from build123d import *

# Parameters (mm, degrees)
F1_DEPTH = 5
F3_D     = 6.6


with BuildPart() as f1:
    # F0 (on Front) → F1 (new body)
    with BuildSketch(Plane.XZ):
        Polygon((-250, 300), (-310, 300), (-310, -300), (310, -300), (310, -100), align=None)
    extrude(amount=F1_DEPTH)

    # F3 (through all)
    with Locations(Plane.XZ.offset(5)):
        with Locations((-125, -285), (0, -285), (125, -285)):
            Hole(F3_D / 2)


solid = f1.part
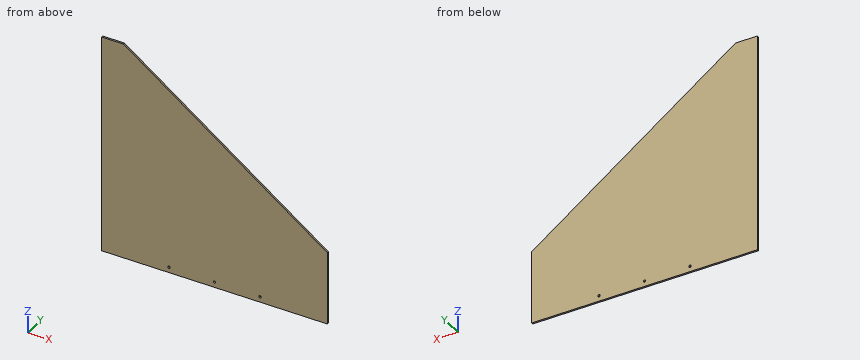
CAD build for the part. Positions are in the model's coordinates, mm. Round coordinates to 2 decimals unless told otherwise and drop trailing zeros. Loops run counter-clockwise (first coordinate to the right, second up) from the corner with the lowest first, then second, coordinate; pieces in that order, holes last.
(1) Wall check: line 1 along X through (y, z) = (-3.05, -285); line 2 along Z through (x, y) = (0, -2.7); line 3 along Z through (x, y) = (125, -2.2). Give the ranges that are in metal, low to high.
(2) Cut at C-C (x = -207). Give the cut face in (y, z).
(3) Drop flat-ended pins along their axis: pin 1 (1.5 mm diameter, centred on x = 11, y = -1, fed in from +Z); pin 2 (1 mm diameter, centred on x = 48, z = -230, fed in from +Y). Give the stop position or say it passes through.
(4) Cut at B-B (z = 236.5). Give the cut face in (x, y).
(5) Cut at A-A (y = -1.6). Give the cut face in (x, z), plus the area to 3 significant figures.
Findings below:
1. line 1: x = -310 to -128.3, -121.7 to -3.3, 3.3 to 121.7, 128.3 to 310
1. line 2: z = -300 to -288.3, -281.7 to 121.43
1. line 3: z = -300 to -288.3, -281.7 to 32.14
2. outline: (-5, -300) - (0, -300) - (0, 269.29) - (-5, 269.29) - close
3. pin 1: stops at z = 114.11
3. pin 2: stops at y = 0
4. outline: (-310, -5) - (-161.1, -5) - (-161.1, 0) - (-310, 0) - close
5. outline: (-310, -300) - (310, -300) - (310, -100) - (-250, 300) - (-310, 300) - close; hole circle Ø6.6 at (-125, -285); hole circle Ø6.6 at (0, -285); hole circle Ø6.6 at (125, -285)
5. area: 260,000 mm2
